Build history of the part. All positions in model axes, mm. Give positions to 0.01 mm unless a question says otherwise; leave off trailing zeros. Write each loop counter-clockwise with the first axis right and the second up, starting at its lowest first coordinate (ties: lowest second). Pieces come first, ordered by that corner, then holes. Notation, with made-up numbers: M 88.25,39.25 L 130.25,39.25 A20 ccw 130.25,77.25 Z; hole C -39.5,-12.75 d6. An arc over 180 degrees is marked long. Return JSON: item names as keys, results as strings. Group by question number.
Q1. Wall check: probe 1 along Y at (x, z) = (0, 32); probe 2 along X at (y, z) = (16, 5); probe 3 along Y at (x, z) = (3.5, 37). Give the ranges that are in metal, low to high.
Q2. Band-saw the part on C-C, the plane z = 40.5. Give the cut face in (x, y).
Q3. Flat gauge pins, fed straight in: pin 1 Ø10 at (y, z) = (-26, 34) entering from -X; pin 2 Ø1 at (x, z) = (-19.5, 51) entering from +Y; pin 3 Ø6 at (y, z) = (31, 39) entering from -X. Where does each tip first touch, or does it go through?
Q4. Band-saw the part on A-A, the plane x = 0. Give the cut face in (y, z), then the cut area to 3 significant figures.
from build123d import *

# Parameters (mm, degrees)
SKETCH2_R           = 44.45
BOSS_EXTRUDE1_DEPTH = 76.2
SHELL1_T            = -2.54
SKETCH3_R           = 41.91
CUT_EXTRUDE1_DEPTH  = 76.2


with BuildPart() as part:
    # Sketch2 → Boss-Extrude1 (new body)
    with BuildSketch(Plane.XY):
        with Locations(Location((0, 0, 0), (0, 0, 180))):
            Circle(SKETCH2_R)
    extrude(amount=BOSS_EXTRUDE1_DEPTH)

    # Shell1
    shell1_openings = [part.faces().sort_by_distance(p)[0] for p in [
        (0, 0, 0),
    ]]
    offset(amount=SHELL1_T, openings=shell1_openings, kind=Kind.INTERSECTION)

    # Sketch3 → Cut-Extrude1 (cut)
    with BuildSketch(Plane(origin=(0, 0, 73.66), x_dir=(-1, 0, 0), z_dir=(0, 0, -1))):
        Circle(SKETCH3_R)
    extrude(amount=-CUT_EXTRUDE1_DEPTH, mode=Mode.SUBTRACT)


solid = part.part
From the geometry:
{
 "1": {"probe 1": "y = -44.45 to -41.91, 41.91 to 44.45", "probe 2": "x = -41.47 to -38.74, 38.74 to 41.47", "probe 3": "y = -44.31 to -41.76, 41.76 to 44.31"},
 "2": {"outline": "C 0,0 d88.9; hole C 0,0 d83.82"},
 "3": {"pin 1": "stops at x = -39.18", "pin 2": "stops at y = 40.18", "pin 3": "stops at x = -34.52"},
 "4": {"outline": "M -44.45,0 L -41.91,0 L -41.91,76.2 L -44.45,76.2 Z; M 41.91,0 L 44.45,0 L 44.45,76.2 L 41.91,76.2 Z", "area": "387 mm^2"}
}
